For this review, take the finished solid that the model builds, in its own axes (mm). A direction names the side the tool comes from. Coordinates: 2 decimals unless noted, no trailing zeros. Write each loop counter-clockwise with the first axis right and the second up, starting at its lowest first coordinate (ties: lowest second). Pieces come first, ordered by that corner, then holes.
```python
from build123d import *

# Parameters (mm, degrees)
F0_W     = 32.004
F0_H     = 16.002
F1_DEPTH = 5.0038
F2_R     = 2.3495
F3_DEPTH = 1.8542
F4_W     = 29.0068
F4_H     = 13.0048
F4_R     = 3.2512
F4_R_2   = 2.4003
F5_DEPTH = 3.5052
F6_SIZE  = 0.254


with BuildPart() as f1:
    # F0 (on Top) → F1 (new body)
    with BuildSketch(Plane.XY):
        Rectangle(F0_W, F0_H)
    extrude(amount=F1_DEPTH)

    # F2 (on face) → F3 (join)
    with BuildSketch(Plane.XY.offset(5.0038)):
        with Locations((-12.0904, 4.0894)):
            Circle(F2_R)
        with Locations((-12.0904, -3.9116)):
            Circle(F2_R)
        with Locations((-4.0894, 4.0894)):
            Circle(F2_R)
        with Locations((-4.0894, -3.9116)):
            Circle(F2_R)
        with Locations((3.9116, 4.0894)):
            Circle(F2_R)
        with Locations((3.9116, -3.9116)):
            Circle(F2_R)
        with Locations((11.9126, 4.0894)):
            Circle(F2_R)
        with Locations((11.9126, -3.9116)):
            Circle(F2_R)
    extrude(amount=F3_DEPTH)

    # F4 (on face) → F5 (cut)
    with BuildSketch(Plane(origin=(0, 0, 0), x_dir=(1, 0, 0), z_dir=(0, 0, -1))):
        Rectangle(F4_W, F4_H)
        with Locations((-8.001, 0)):
            Circle(F4_R, mode=Mode.SUBTRACT)
        Circle(F4_R, mode=Mode.SUBTRACT)
        with Locations((8.001, 0)):
            Circle(F4_R, mode=Mode.SUBTRACT)
        with Locations((-8.001, 0)):
            Circle(F4_R_2)
        with Locations((8.001, 0)):
            Circle(F4_R_2)
        Circle(F4_R_2)
    extrude(amount=-F5_DEPTH, mode=Mode.SUBTRACT)

    # F6
    f6_edges = [f1.edges().sort_by_distance(p)[0] for p in [
        (-14.4399, 4.0894, 6.858),
        (-14.4399, -3.9116, 6.858),
        (-6.4389, -3.9116, 6.858),
        (-6.4389, 4.0894, 6.858),
        (1.5621, 4.0894, 6.858),
        (1.5621, -3.9116, 6.858),
        (9.5631, -3.9116, 6.858),
        (9.5631, 4.0894, 6.858),
    ]]
    chamfer(f6_edges, length=F6_SIZE)


solid = f1.part
```
Q1. Tool access review of faces 5 (the flat face through (12, 4, 6.858)), 6 (the cylindrical face through (3.61, -1.58, 5.79)), 7 (the flat face through (14.503, 0, 2)): name each direction out of +Z, -Z, +X, -X, +Y, -Y from which nothing blocks a thin tool from reaching the whole face with its end or side.
Ans:
face 5: +Z, +X, -X, +Y, -Y
face 6: +Z
face 7: -Z
Q2. Add section B-B (z = 5.5). State the section outline as (x, y) points.
Ans:
outline: circle Ø4.7 at (-12.09, -3.91); circle Ø4.7 at (-12.09, 4.09); circle Ø4.7 at (-4.09, -3.91); circle Ø4.7 at (-4.09, 4.09); circle Ø4.7 at (3.91, -3.91); circle Ø4.7 at (3.91, 4.09); circle Ø4.7 at (11.91, -3.91); circle Ø4.7 at (11.91, 4.09)
Q3. For probe 1 along Y at (x, z) = (0, 1.7); probe 2 along Y at (x, z) = (9, 2.5); probe 3 along Z at (x, y) = (14, 5.5), list the stretches that pass through material, from the lowest coordinate up.
Ans:
probe 1: y = -8 to -6.5, -3.25 to -2.4, 2.4 to 3.25, 6.5 to 8
probe 2: y = -8 to -6.5, -3.09 to -2.18, 2.18 to 3.09, 6.5 to 8
probe 3: z = 3.51 to 5
Q4. Add section C-C (x = 0). State the section outline as (y, z) points.
Ans:
outline: (-8, 0) - (-6.5, 0) - (-6.5, 3.51) - (-3.25, 3.51) - (-3.25, 0) - (-2.4, 0) - (-2.4, 3.51) - (2.4, 3.51) - (2.4, 0) - (3.25, 0) - (3.25, 3.51) - (6.5, 3.51) - (6.5, 0) - (8, 0) - (8, 5) - (-8, 5) - close
Q5. Add section A-A (z = 2.25). State the section outline as (x, y) points.
Ans:
outline: (-16, -8) - (16, -8) - (16, 8) - (-16, 8) - close; circle Ø6.5 at (-8, 0); circle Ø6.5 at (0, 0); circle Ø6.5 at (8, 0); hole (-14.5, -6.5) - (14.5, -6.5) - (14.5, 6.5) - (-14.5, 6.5) - close; hole circle Ø4.8 at (-8, 0); hole circle Ø4.8 at (0, 0); hole circle Ø4.8 at (8, 0)
Q6. Clearance check with flat-ended pins moving along their axes: pin 1 Ø1.4 at (x, y) = (8.5, 0.5) entering from -Z; pin 2 Ø5.5 at (x, y) = (-8.001, 0) entering from +Z; pin 3 Ø1 at (x, z) = (-1, 6) entering from +Y. State where each tip first meets the part, or that it passes through.
Ans:
pin 1: stops at z = 3.51
pin 2: stops at z = 5
pin 3: passes through
Q7. Draft analysis for pull direction X (two halves, no side actions). For faces 1 (the flat face through (-16.002, 0, 2)), 2 (the cylindrical face through (6.23, -1.62, 1.73)), 3 (the flat face through (-4, 4, 6.858)), 4 (the flat face through (16.002, 0, 2)), state which applies: +X half, -X half, draft (parallel to the pull), parting line (faces both ways), or undercut.
Ans:
face 1: -X half
face 2: undercut
face 3: draft
face 4: +X half
